from build123d import *

# Parameters (mm, degrees)
F0_W      = 38.1
F0_H      = 38.1
F1_DEPTH  = 38.1
F6_DEPTH  = 38.1
F9_DEPTH  = 38.1
F10_W     = 25.4
F10_H     = 7.62
F11_DEPTH = 38.1


with BuildPart() as f1:
    # F0 (on Front) → F1 (new body)
    with BuildSketch(Plane.XZ):
        with Locations((19.05, 19.05)):
            Rectangle(F0_W, F0_H)
    extrude(amount=F1_DEPTH)

    # F5 (on offset) → F6 (cut)
    with BuildSketch(Plane.YZ.offset(38.1)):
        Polygon((-6.35, 38.1), (-31.75, 38.1), (-26.67, 16.8241550819), (-21.59, 28.575), (-16.51, 28.575), (-11.43, 16.8241550819), align=None)
        Polygon((-31.75, 0), (-38.1, 38.1), (-38.1, 0), align=None)
        Polygon((-19.05, 15.875), (-25.4, 0), (-22.9262417018, 0), (-19.05, 0), (-12.7, 0), align=None)
        Polygon((0, 0), (0, 38.1), (-6.35, 0), align=None)
    extrude(amount=-F6_DEPTH, mode=Mode.SUBTRACT)

    # F8 (on face) → F9 (cut)
    with BuildSketch(Plane.XZ.offset(38.1)):
        Polygon((0, 37.9714828326), (0, 0), (6.3321403529, 37.9928421172), align=None)
        Polygon((11.43, 22.225), (6.35, 0), (31.75, 0), (26.67, 22.225), (21.59, 9.525), (16.51, 9.525), align=None)
        Polygon((25.382841226, 38.057103065), (12.7342250661, 38.0144373348), (19.05, 22.225), align=None)
        Polygon((31.7535679155, 38.0785925072), (38.1, 0), (38.1, 38.1), align=None)
    extrude(amount=-F9_DEPTH, mode=Mode.SUBTRACT)

    # F10 (on offset) → F11 (cut)
    with BuildSketch(Plane.XY.offset(38.1)):
        with Locations((25.4, -11.43)):
            Rectangle(F10_W, F10_H)
        with Locations((12.7, -26.67)):
            Rectangle(F10_W, F10_H)
    extrude(amount=-F11_DEPTH, mode=Mode.SUBTRACT)


solid = f1.part
Verification items for the finished model (mm, model axes). A direction names the side the tool comes from. Give positions to 0.01 mm unless a question says otherwise; leave off trailing zeros. Order: outer loops, then holes, each group sorted by start corner. A loop starts at its lowest first (then second) coordinate and runs counter-clockwise, first axis right, second up. Notation, with made-up numbers: M 84,84.25 L 114,84.25 A24 ccw 114,123.25 Z; hole C -11,6.5 d2. An arc over 180 degrees is marked long. Use one line per item in the form item = value. Start each with the question number.
Q1. Scan lines: line 1 along Y through (x, z) = (28.5, 14.5); line 2 along Y through (x, z) = (33, 15.5); line 3 along X through (y, z) = (-16.5, 19). Record each from-to range of solid material in increasing order. Write a range as [from, to].
Q2. Access from +Z, -Z, +X, -X, +Y, -Y to the whole of each face (thin tool, end or side, straight path). Record for faces 1 (the flat face through (3, -9, 0)), 2 (the flat face through (16, -22.86, 18)), 3 (the flat face through (14, -32.4, 15.8)), 4 (the flat face through (19.121, -18.044, 13.361)), 5 (the flat face through (12.083, -8.526, 28.988)).
Q3. Section check A-A (z = 28). Enter the section's corners in (x, y), then the cut area to 3 significant figures.
Q4. Section check C-C (z = 34). Enter the section's corners in (x, y), then the cut area to 3 significant figures.
Q5. Section check B-B (y = -5.5). Enter the section's corners in (x, z) (3 decimals).
Q6. Mould release check, pull along X, two halves, no side actions. Record for faces 6 (the flat face through (5.06, -15.83, 7.83)), 7 (the flat face through (22.17, -4.71, 30.03)), 8 (the flat face through (20.302, -19.103, 25.356)), 9 (the flat face through (34.177, -4.711, 23.537)): +X half, -X half, draft (parallel to the pull), parting line (faces both ways), or undercut.
Q7. Go/stop test with flat-tipped pins: pin 1 Ø8 at (y, z) = (-25, 13.5) entering from -X; pin 2 Ø4 at (x, y) = (27.5, -19) entering from +Z (3 decimals); pin 3 Ø1 at (x, y) = (13, -28) entering from +Z; pin 4 Ø3.5 at (y, z) = (-28.5, 23) entering from -X. Record where each tip stops, or that it passes through.
Evaluation:
q1.line_1 = [-34.17, -19.6], [-18.5, -15.24], [-7.62, -3.93]
q1.line_2 = [-34.33, -19.2], [-18.9, -15.24], [-7.62, -3.77]
q1.line_3 = [3.17, 10.69], [12.72, 25.38], [27.41, 34.93]
q2.face_1 = -Z, +X, -X, +Y, -Y
q2.face_2 = +Z, -Z, -X
q2.face_3 = -Z, +Y, -Y
q2.face_4 = -Z, +X, -X
q2.face_5 = +Z, +X, -X
q3.outline = M 4.67,-36.42 L 16.74,-36.42 L 16.74,-30.48 L 4.67,-30.48 Z; M 4.67,-21.84 L 16.74,-21.84 L 16.74,-16.26 L 4.67,-16.26 Z; M 4.67,-8.76 L 12.7,-8.76 L 12.7,-7.62 L 16.74,-7.62 L 16.74,-1.68 L 4.67,-1.68 Z; M 21.36,-36.42 L 33.43,-36.42 L 33.43,-29.34 L 25.4,-29.34 L 25.4,-30.48 L 21.36,-30.48 Z; M 21.36,-21.84 L 33.43,-21.84 L 33.43,-16.26 L 21.36,-16.26 Z; M 21.36,-7.62 L 33.43,-7.62 L 33.43,-1.68 L 21.36,-1.68 Z
q3.area = 440 mm2
q4.outline = M 5.67,-37.42 L 14.34,-37.42 L 14.34,-30.77 L 5.67,-30.77 Z; M 5.67,-7.33 L 14.34,-7.33 L 14.34,-0.68 L 5.67,-0.68 Z; M 23.76,-37.42 L 32.43,-37.42 L 32.43,-30.77 L 23.76,-30.77 Z; M 23.76,-7.33 L 32.43,-7.33 L 32.43,-0.68 L 23.76,-0.68 Z
q4.area = 231 mm2
q5.outline = M 0,37.971 L 6.332,37.993 L 0.85,5.1 L 7.516,5.1 L 11.43,22.225 L 16.51,9.525 L 21.59,9.525 L 26.67,22.225 L 30.584,5.1 L 37.25,5.1 L 31.754,38.079 L 38.1,38.1 L 0,38.1 Z; hole M 12.734,38.014 L 19.05,22.225 L 25.383,38.057 Z
q6.face_6 = draft
q6.face_7 = undercut
q6.face_8 = undercut
q6.face_9 = +X half
q7.pin_1 = 1.69
q7.pin_2 = 28.575
q7.pin_3 = through
q7.pin_4 = 25.4
